For this review, take the finished solid that the model builds, in its own axes (mm). Give positions to 0.01 mm unless a question says otherwise; leave off trailing zeros. Order: outer loops, then holes, each group sorted by start corner. A loop starts at its lowest first (then second) coordinate and runs counter-clockwise, first axis right, second up. Notation, with made-up numbers: (-36, -10) - (-25, -10) arc R34 ccw to (-25, 23) - close; hole circle Ø5 at (-38, -11). An arc over 180 degrees is marked (long way). Answer as a JSON object with one key per item and string values. Group by question number.
from build123d import *

# Parameters (mm, degrees)
IZIM1_W               = 200
IZIM1_H               = 40
TABAN_FLAN_1_DEPTH    = 4
IZIM6_R               = 7.75
IZIM6_R_2             = 8
KES_EKSTR_ZYON1_DEPTH = 10
RADYUS1_R             = 10


# Sheet-metal steps are written as plain solids
with BuildPart() as part:
    # Çizim1 → Taban-Flanş1 (new body)
    with BuildSketch(Plane.XY):
        Rectangle(IZIM1_W, IZIM1_H)
    extrude(amount=-TABAN_FLAN_1_DEPTH)

    # Çizim6 → Kes-Ekstrüzyon1 (cut)
    with BuildSketch(Plane.XY):
        with Locations((-85, 0)):
            Circle(IZIM6_R)
        with Locations((50, 0)):
            Circle(IZIM6_R_2)
    extrude(amount=-KES_EKSTR_ZYON1_DEPTH, mode=Mode.SUBTRACT)

    # Radyus1
    radyus1_edges = [part.edges().sort_by_distance(p)[0] for p in [
        (-100, -20, -2),
        (-100, 20, -2),
    ]]
    fillet(radyus1_edges, radius=RADYUS1_R)


solid = part.part
1) Consider section D-D (x = 50). Give the boundary of the cut face in (y, z).
2) For line 1 (Y direction, x = -85, z = -3.05); line 2 (X direction, y = -1, z = -3.35); line 3 (Y direction, x = 50, z = -1.2), list the stretches that pass through material, from the lowest coordinate up.
3) Consider section B-B (z = -3.4). Give the boundary of the cut face in (x, y).
4) Consider section C-C (y = -6). Give the boundary of the cut face in (x, z), plus the area to 3 significant figures.
5) Consider section A-A (x = -85). Give the boundary of the cut face in (y, z).
6) For pin 1 (21 mm diameter, centred on x = 50, y = 0, fed in from -Z), flat-tipped, find the tip position at first contact; note if it passes through.
Result set:
{
 "1": {"outline": "(-20, -4) - (-8, -4) - (-8, 0) - (-20, 0) - close; (8, -4) - (20, -4) - (20, 0) - (8, 0) - close"},
 "2": {"line 1": "y = -20 to -7.75, 7.75 to 20", "line 2": "x = -100 to -92.69, -77.31 to 42.06, 57.94 to 100", "line 3": "y = -20 to -8, 8 to 20"},
 "3": {"outline": "(-100, -10) arc R10 ccw to (-90, -20) - (100, -20) - (100, 20) - (-90, 20) arc R10 ccw to (-100, 10) - close; hole circle Ø15.5 at (-85, 0); hole circle Ø16 at (50, 0)"},
 "4": {"outline": "(-100, -4) - (-89.91, -4) - (-89.91, 0) - (-100, 0) - close; (-80.09, -4) - (44.71, -4) - (44.71, 0) - (-80.09, 0) - close; (55.29, -4) - (100, -4) - (100, 0) - (55.29, 0) - close", "area": "718 mm2"},
 "5": {"outline": "(-20, -4) - (-7.75, -4) - (-7.75, 0) - (-20, 0) - close; (7.75, -4) - (20, -4) - (20, 0) - (7.75, 0) - close"},
 "6": {"pin 1": "stops at z = -4"}
}
